Build history of the part. All positions in model axes, mm. A direction names the side the tool comes from. Round coordinates to 2 decimals unless told otherwise and drop trailing zeros. Loops run counter-clockwise (first coordinate to the right, second up) from the corner with the lowest first, then second, coordinate; pieces in that order, holes last. Notation, with made-up numbers: (-14.75, 2.25) - (22.25, 2.25) arc R13 ccw to (22.25, 11.25) - close; hole circle Ø4 at (63, 30). An arc over 180 degrees is marked (long way). Use a Markdown table: item, result.
from build123d import *

# Parameters (mm, degrees)
F2_R     = 1.5875
F3_DEPTH = 11.1125
F4_R     = 4.7625
F5_DEPTH = 9.525


with BuildPart() as f1:
    # F0 (on Front) → F1 (revolve)
    with BuildSketch(Plane.XZ):
        Polygon((0, 50.45817), (0, 0), (6.916383, 0), (31.75, 15.876247), (21.236976, 32.320713), (7.545146, 23.567463), (7.545146, 50.45817), align=None)
    revolve(axis=Axis((0, 0, 25.229085), (0, 0, -1)))

    # F2 (on face) → F3 (cut)
    with BuildSketch(Plane(origin=(0, 0, 0), x_dir=(1, 0, 0), z_dir=(0, 0, -1))):
        Circle(F2_R)
    extrude(amount=-F3_DEPTH, mode=Mode.SUBTRACT)

    # F4 (on face) → F5 (cut)
    with BuildSketch(Plane.XY.offset(50.45817)):
        Circle(F4_R)
    extrude(amount=-F5_DEPTH, mode=Mode.SUBTRACT)


solid = f1.part
Q1. Pull direction Y, two halves, no side cores. Call faces 1 (the face through (-1.78, 8.01, 23.99)), 2 (the face through (-2.831, -21.562, 31.522)), 3 (the face through (0, 5, 50.458)): pulls with the +Y half, pulls with the -Y half, needs draft (parallel to the pull), parting line crosses it, or undercut.
Results found:
| item | result |
|---|---|
| face 1 | undercut |
| face 2 | parting line crosses it |
| face 3 | needs draft |
Q2. Cut at A-A, the plane y = 0. List the corners of the cut face in (x, z), plus the area to 3 significant figures.
Results found:
| item | result |
|---|---|
| outline | (-31.75, 15.88) - (-6.92, 0) - (-1.59, 0) - (-1.59, 11.11) - (1.59, 11.11) - (1.59, 0) - (6.92, 0) - (31.75, 15.88) - (21.24, 32.32) - (7.55, 23.57) - (7.55, 50.46) - (4.76, 50.46) - (4.76, 40.93) - (-4.76, 40.93) - (-4.76, 50.46) - (-7.55, 50.46) - (-7.55, 23.57) - (-21.24, 32.32) - close |
| area | 1,510 mm2 |
Q3. Drop flat-ended pins along their axis: pin 1 (4 mm diameter, centred on x = -12.5, y = 25, fed in from +Z); pin 2 (2 mm diameter, centred on y = 9, z = 40.5, fed in from -X); pin 3 (4 mm diameter, centred on x = 0, y = 0, fed in from +Z); pin 4 (1.5 mm diameter, centred on x = -19.5, y = 10.5, fed in from +Z). Give the stop position or say it passes through.
Results found:
| item | result |
|---|---|
| pin 1 | stops at z = 24.95 |
| pin 2 | passes through |
| pin 3 | stops at z = 40.93 |
| pin 4 | stops at z = 32.07 |
Q4. Which spindle directions (+Z, -Z, +X, -X, +Y, -Y) get a long thin tool onto all of the face, cutting with end or side? Do faces 4 (the face through (0, 0, 11.112)), 5 (the face through (0, -2, 0)), 6 (the face through (-3.78, -2.9, 45.76)). Say none if no direction does.
Results found:
| item | result |
|---|---|
| face 4 | -Z |
| face 5 | -Z, +X, -X, +Y, -Y |
| face 6 | +Z |
Q5. Cut at D-D, the plane z = 39.5. List the corners of the cut face in (x, y).
Results found:
| item | result |
|---|---|
| outline | circle Ø15.09 at (0, 0) |
Q6. Cut at C-C, the plane z = 27. List the corners of the cut face in (x, y).
Results found:
| item | result |
|---|---|
| outline | circle Ø49.28 at (0, 0); circle Ø15.09 at (0, 0); hole circle Ø25.83 at (0, 0) |
Q7. Probe line 1 (Y direction, x = 0, z = 46); line 2 (X direction, y = 0, z = 2); line 3 (X direction, y = 0, z = 8.5). List the from-to ranges inside material, lowest first.
Results found:
| item | result |
|---|---|
| line 1 | y = -7.55 to -4.76, 4.76 to 7.55 |
| line 2 | x = -10.04 to -1.59, 1.59 to 10.04 |
| line 3 | x = -20.21 to -1.59, 1.59 to 20.21 |
